```python
from build123d import *

# Parameters (mm, degrees)
F0_W           = 27.94
F0_H           = 50.8
F1_DEPTH       = 33.02
F2_W           = 7.9375
F2_H           = 50.8
F3_DEPTH       = 7.62
F4_W           = 15.875
F4_H           = 7.9375
F5_DEPTH       = 7.62
F6_W           = 15.6845
F6_H           = 7.9375
F7_DEPTH       = 25.4
F8_W           = 9.8425
F8_H           = 16.35125
F9_DEPTH       = 33.02
F11_DEPTH      = 27.941
F13_DEPTH      = 25.401
F13_DEPTH_BACK = 25.4
F14_W          = 9.8425
F14_H          = 7.62
F15_DEPTH      = 34.44975
F17_DEPTH      = 34.44975


with BuildPart() as f1:
    # F0 (on Top) → F1 (new body)
    with BuildSketch(Plane.XY):
        Rectangle(F0_W, F0_H)
    extrude(amount=F1_DEPTH)

    # F2 (on face) → F3 (cut)
    with BuildSketch(Plane(origin=(0, 0, 0), x_dir=(1, 0, 0), z_dir=(0, 0, -1))):
        with Locations((-4.92125, 0)):
            Rectangle(F2_W, F2_H)
    extrude(amount=-F3_DEPTH, mode=Mode.SUBTRACT)

    # F4 (on face) → F5 (cut, through all)
    with BuildSketch(Plane(origin=(0, 0, 0), x_dir=(1, 0, 0), z_dir=(0, 0, -1))):
        with Locations((6.985, 0)):
            Rectangle(F4_W, F4_H)
    extrude(amount=-F5_DEPTH, mode=Mode.SUBTRACT)

    # F6 (on face) → F7 (cut, through all)
    with BuildSketch(Plane(origin=(0, 0, 7.62), x_dir=(1, 0, 0), z_dir=(0, 0, -1))):
        with Locations((6.12775, 0)):
            Rectangle(F6_W, F6_H)
    extrude(amount=-F7_DEPTH, mode=Mode.SUBTRACT)

    # F8 (on face) → F9 (cut, through all)
    with BuildSketch(Plane(origin=(0, 0, 0), x_dir=(1, 0, 0), z_dir=(0, 0, -1))):
        with Locations((9.04875, -17.224375)):
            Rectangle(F8_W, F8_H)
        with Locations((9.04875, 17.224375)):
            Rectangle(F8_W, F8_H)
    extrude(amount=-F9_DEPTH, mode=Mode.SUBTRACT)

    # F10 (on face) → F11 (cut, through all)
    with BuildSketch(Plane(origin=(-13.97, 0, 0), x_dir=(0, -1, 0), z_dir=(-1, 0, 0))):
        Polygon((-25.4, 12.7), (-9.04875, 33.02), (-25.4, 33.02), align=None)
        Polygon((25.4, 33.02), (9.04875, 33.02), (25.4, 12.7), align=None)
    extrude(amount=-F11_DEPTH, mode=Mode.SUBTRACT)

    # F12 (on Front) → F13 (cut, two sides)
    with BuildSketch(Plane.XZ) as f13_sk:
        Polygon((-6.7945, 33.02), (-13.97, 33.02), (-13.97, 12.7), align=None)
    extrude(amount=-F13_DEPTH, mode=Mode.SUBTRACT)
    extrude(f13_sk.sketch, amount=F13_DEPTH_BACK, mode=Mode.SUBTRACT)

    # F14 (on face) → F15 (cut, through all)
    with BuildSketch(Plane(origin=(0, 9.04875, 0), x_dir=(-1, 0, 0), z_dir=(0, 1, 0))):
        with Locations((-9.04875, 3.81)):
            Rectangle(F14_W, F14_H)
    extrude(amount=-F15_DEPTH, mode=Mode.SUBTRACT)

    # F16 (on face) → F17 (cut, through all)
    with BuildSketch(Plane.XZ.offset(9.04875)):
        Polygon((13.97, 33.02), (4.1275, 33.02), (13.97, 7.62), align=None)
    extrude(amount=-F17_DEPTH, mode=Mode.SUBTRACT)


solid = f1.part
```
The listing builds one solid part. Answer for the finished solid, in the listing's coordinates (mm). A direction names the side the tool comes from. Round coordinates to 2 decimals unless told otherwise and drop trailing zeros. Write each loop counter-clockwise with the first axis right and the second up, starting at its lowest first coordinate (ties: lowest second). Pieces come first, ordered by that corner, then holes. Notation, with made-up numbers: (4.25, 75.5) -> (38.25, 75.5) arc R28 ccw to (38.25, 106.5) -> close; hole circle Ø3 at (-23.5, -18.75). An arc over 180 degrees is marked (long way). Use CSV: the item, a comma, the result in double quotes. Start each with the question number.
(1) Section A-A on x = 3 is taken. Give the vertices of the cut face in (y, z), then the cut area to 3 significant figures.
(2) Each of these flat-tipped pins is pushed along its axis until it touches: pin 1 (3 mm diameter, centred on x = 8, z = 22.5, fed in from +Y); pin 2 (6.5 mm diameter, centred on y = 0, z = 24, fed in from +X); pin 3 (4.5 mm diameter, centred on x = 6, z = 21.5, fed in from -Y). Where does it stop, or does it pass through?
(3) Section C-C on z = 13.5 is taken. Give the vertices of the cut face in (x, y), then the cut area to 3 significant figures.
(4) Which of the six approach directions +Z, -Z, +X, -X, +Y, -Y give full straight-line access (tool end or side, diameter ignored) to faces 1 (the face through (-8.89, 0, 4)), 2 (the face through (9, -6, 7.62)), 3 (the face through (8, -9.049, 17))?
(5) Section D-D on x = -3.25 is taken. Give the vertices of the cut face in (y, z), then the cut area to 3 significant figures.
(6) Section B-B on y = -8.5 is taken. Give the vertices of the cut face in (x, z).
(7) The mould has two halves that part along Y. Classify faces 4 (the face through (-1.715, 0, 20)), 5 (the face through (2, -15, 0)), 6 (the face through (4, -3.969, 16)), 7 (the face through (8, 9.049, 17)): released by +Y, released by -Y, zero draft, split by the parting line, or undercut.
(8) Consider L1, parallel to X at y = 4, z = 7; L2, parallel to Y at x = 10.75, z = 15.5; L3, parallel to X at y = 9.5, z = 11.5. Determine where each line is inside the solid, lowest interval first. Write a range as from..to.
A:
1,outline,"(-25.4, 0) -> (-3.97, 0) -> (-3.97, 33.02) -> (-9.05, 33.02) -> (-25.4, 12.7) -> close; (3.97, 0) -> (25.4, 0) -> (25.4, 12.7) -> (9.05, 33.02) -> (3.97, 33.02) -> close"
1,area,"1,080 mm²"
2,pin 1,"stops at y = 9.05"
2,pin 2,"stops at x = -1.71"
2,pin 3,"stops at y = -19.32"
3,outline,"(-13.69, -24.76) -> (4.13, -24.76) -> (4.13, -9.05) -> (11.69, -9.05) -> (11.69, -3.97) -> (-1.71, -3.97) -> (-1.71, 3.97) -> (11.69, 3.97) -> (11.69, 9.05) -> (4.13, 9.05) -> (4.13, 24.76) -> (-13.69, 24.76) -> close"
3,area,"913 mm²"
4,face 1,"-Z, +Y, -Y"
4,face 2,"-Z, +X, +Y, -Y"
4,face 3,"+Z, -Z, +X, -Y"
5,outline,"(-25.4, 7.62) -> (25.4, 7.62) -> (25.4, 12.7) -> (9.05, 33.02) -> (-9.05, 33.02) -> (-25.4, 12.7) -> close"
5,area,"958 mm²"
6,outline,"(-13.97, 0) -> (-8.89, 0) -> (-8.89, 7.62) -> (-0.95, 7.62) -> (-0.95, 0) -> (4.13, 0) -> (4.13, 7.62) -> (13.97, 7.62) -> (4.13, 33.02) -> (-6.79, 33.02) -> (-13.97, 12.7) -> close"
7,face 4,"undercut"
7,face 5,"zero draft"
7,face 6,"undercut"
7,face 7,"released by +Y"
8,L1,"x = -13.97..-8.89, -0.95..4.13"
8,L2,"y = -9.05..-3.97, 3.97..9.05"
8,L3,"x = -13.97..4.13"
